Input: dimensioned drawing with shaded views. Units: mm. Origin: part minimum x, y, z. A direction names the side the tool comes from. Coordinates: 2 decimals unless noted, no trailing zeros. Order: outer loops, then holes, each group sorted by start corner. A loop starts at its lowest first (then second) coordinate and runs counter-clockwise, first axis right, second up.
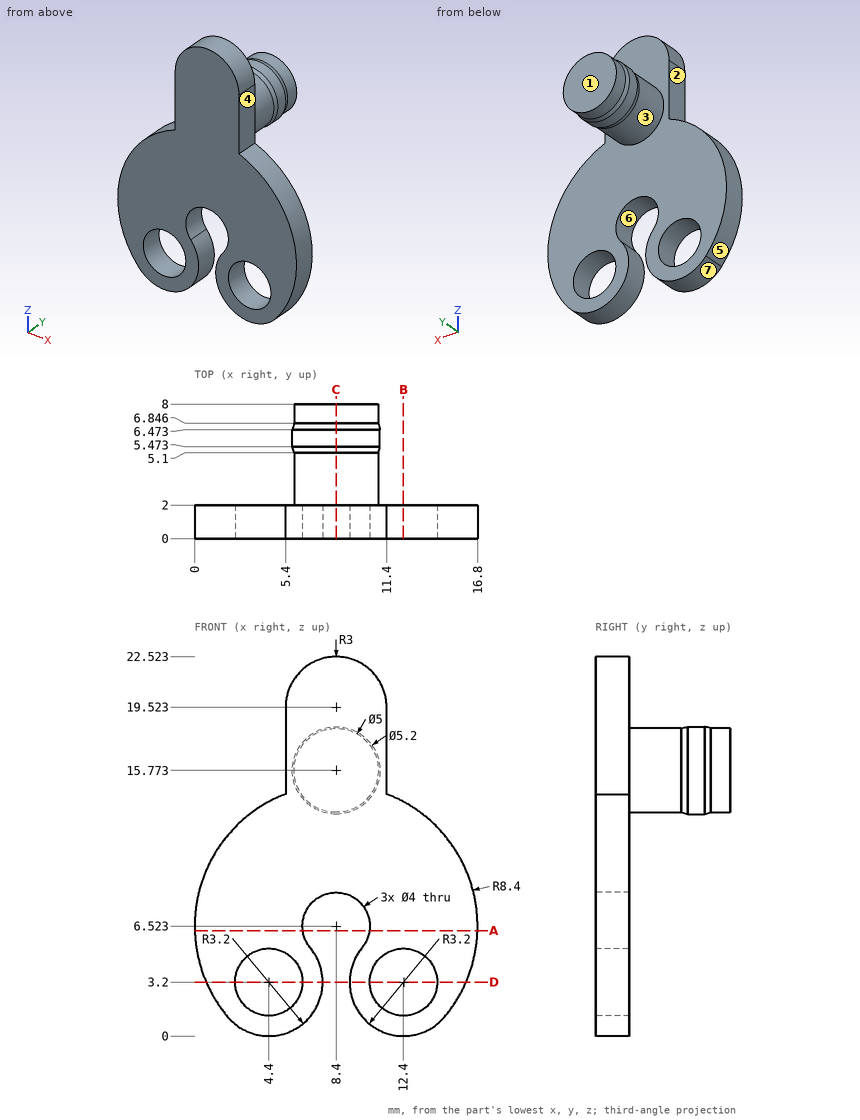
1. Section query D-D, the plane z = 3.2. Output: boundary loops of the cut face in (x, y) (1 decimal).
2. Section query C-C, the plane x = 8.4. Output: boundary loops of the cut face in (y, z).
3. Material intervals for line 1 along X through (y, z) = (1.25, 4); line 2 along X through (y, z) = (1.65, 3.2) (1 decimal); line 3 along Y through (x, z) = (15.5, 7.5), sorted ascending.
4. Section query A-A, the plane z = 6.25. Output: boundary loops of the cut face in (x, y) (1 decimal).
5. Contact query for flat-ended pins moving along their axis: P1, Ø6, axis at x = 4, z = 9, coming from the +Y side; P2, Ø1, axis at y = 1.5, z = 16.5, coming from the -X side; P3, Ø3.5, axis at x = 4.4, z = 3.2, coming from the +Y side; P4, Ø0.6, axis at y = 0.5, z = 17, coming from the +X side. Output: stop coordinate, or through.
6. Access query for the marked faces 1, 2 and 3. Directions: +Z, -Z, +X, -X, +Y, -Y. A direction counts if a zero-diameter tool reaches every point of the face in a straight line with its end or side. Return the directions, or none.
7. Section query B-B, the plane x = 12.4. Output: boundary loops of the cut face in (y, z), plus the area to 3 significant figures.
8. Draft query along Z for the marked faces 4, 5, 6 and 7. Return one class per face: +Z half, -Z half, draft (parallel to the pull), parting line (faces both ways), or undercut.
Answer key:
1. outline: (0.7, 0) - (2.4, 0) - (2.4, 2) - (0.7, 2) - close; (6.4, 0) - (7.6, 0) - (7.6, 2) - (6.4, 2) - close; (9.2, 0) - (10.4, 0) - (10.4, 2) - (9.2, 2) - close; (14.4, 0) - (16.1, 0) - (16.1, 2) - (14.4, 2) - close
2. outline: (0, 8.52) - (2, 8.52) - (2, 13.27) - (5.1, 13.27) - (5.47, 13.17) - (6.47, 13.17) - (6.85, 13.27) - (8, 13.27) - (8, 18.27) - (6.85, 18.27) - (6.47, 18.37) - (5.47, 18.37) - (5.1, 18.27) - (2, 18.27) - (2, 22.52) - (0, 22.52) - close
3. line 1: x = 0.39 to 2.57, 6.23 to 7.5, 9.3 to 10.57, 14.23 to 16.41
3. line 2: x = 0.7 to 2.4, 6.4 to 7.6, 9.2 to 10.4, 14.4 to 16.1
3. line 3: y = 0 to 2
4. outline: (0, 0) - (6.4, 0) - (6.4, 2) - (0, 2) - close; (10.4, 0) - (16.8, 0) - (16.8, 2) - (10.4, 2) - close
5. P1: stops at y = 2
5. P2: stops at x = 5.4
5. P3: passes through
5. P4: stops at x = 11.4
6. face 1: +Z, -Z, +X, -X, +Y
6. face 2: +Z, -X, +Y, -Y
6. face 3: none
7. outline: (0, 0) - (2, 0) - (2, 1.2) - (0, 1.2) - close; (0, 5.2) - (2, 5.2) - (2, 13.91) - (0, 13.91) - close
7. area: 19.8 mm2
8. face 4: draft
8. face 5: parting line
8. face 6: undercut
8. face 7: undercut
